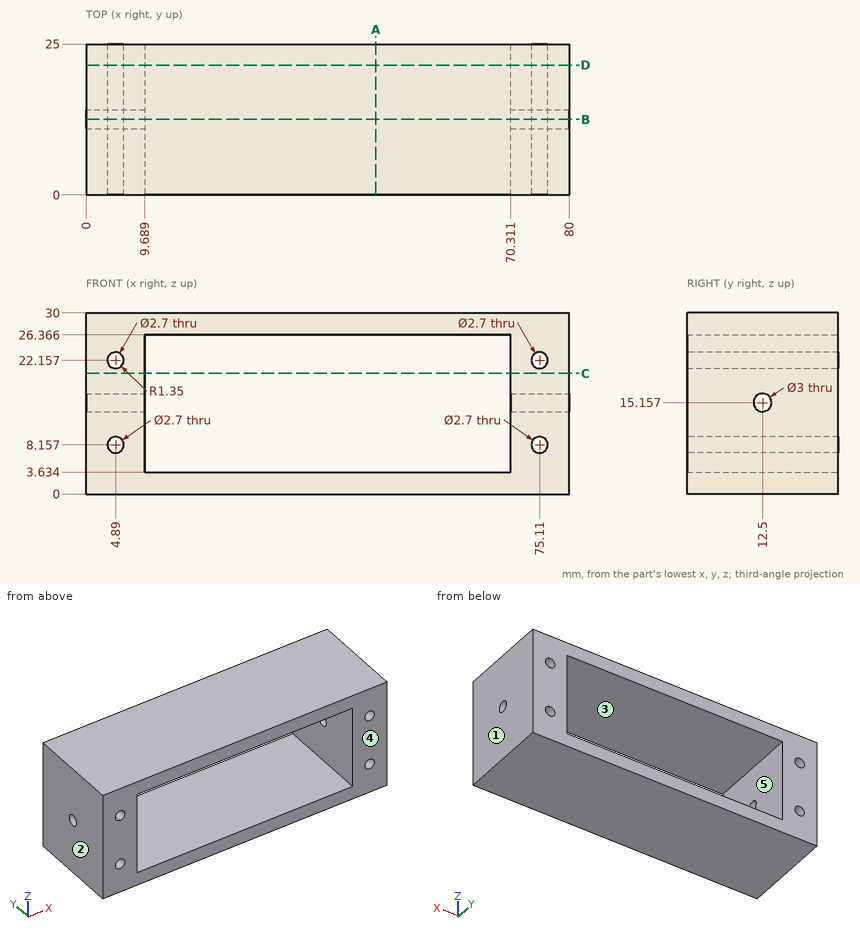
Geometry check sheet. Reference: drawing and pictorial views, mm from the part's lowest x, y, z. A direction names the side the tool comes from. Round coordinates to 2 decimals unless told otherwise and drop trailing zeros. Write each loop counter-clockwise with the first axis right and the second up, starting at its lowest first coordinate (ties: lowest second). Pieces come first, ordered by that corner, then holes. Notation, with made-up numbers: (-30, 80.5) -> (-12, 80.5) arc R25 ccw to (-12, 101.5) -> close; hole circle Ø8 at (43, 32). An arc over 180 degrees is marked (long way). Put each result on its own line as item: value.
1) Release check for a two-part mould opening along X. For the marked faces 1, 2 and 3 record: pulls with the +X half, pulls with the -X half, needs draft (parallel to the pull), parting line crosses it, or undercut.
Recorded:
face 1: pulls with the +X half
face 2: pulls with the -X half
face 3: undercut
2) Cross-section at B-B, the plane y = 12.5. Enter the section's corners in (x, z).
Recorded:
outline: (0, 0) -> (80, 0) -> (80, 13.66) -> (70.31, 13.66) -> (70.31, 3.63) -> (9.69, 3.63) -> (9.69, 13.66) -> (0, 13.66) -> close; (0, 16.66) -> (9.69, 16.66) -> (9.69, 26.37) -> (70.31, 26.37) -> (70.31, 16.66) -> (80, 16.66) -> (80, 30) -> (0, 30) -> close; hole circle Ø2.7 at (4.89, 8.16); hole circle Ø2.7 at (4.89, 22.16); hole circle Ø2.7 at (75.11, 8.16); hole circle Ø2.7 at (75.11, 22.16)
3) Thickness scan on probe 1 along X at (y, z) = (11.5, 4.5); probe 2 along Z at (x, y) = (21, 10.5); probe 3 along Y at (x, z) = (71, 16.5) (1 decimal). Record the ranges inside material, lowest first. Write a range as from..to.
Recorded:
probe 1: x = 0..9.69, 70.31..80
probe 2: z = 0..3.63, 26.37..30
probe 3: y = 0..11.8, 13.2..25
4) Cross-section at A-A, the plane x = 48. Enter the section's corners in (y, z), plus the area to 3 significant figures.
Recorded:
outline: (0, 0) -> (25, 0) -> (25, 3.63) -> (0, 3.63) -> close; (0, 26.37) -> (25, 26.37) -> (25, 30) -> (0, 30) -> close
area: 182 mm2
5) Access from +Z, -Z, +X, -X, +Y, -Y to the whole of each face (thin tool, end or side, straight path). Record for the marked faces 4 and 5.
Recorded:
face 4: +Z, -Z, +X, -X, -Y
face 5: +Y, -Y
6) Cross-section at D-D, the plane y = 21.5. Enter the section's corners in (x, z), plus the area to 3 significant figures.
Recorded:
outline: (0, 0) -> (80, 0) -> (80, 30) -> (0, 30) -> close; hole circle Ø2.7 at (4.89, 8.16); hole circle Ø2.7 at (4.89, 22.16); hole (9.69, 3.63) -> (70.31, 3.63) -> (70.31, 26.37) -> (9.69, 26.37) -> close; hole circle Ø2.7 at (75.11, 8.16); hole circle Ø2.7 at (75.11, 22.16)
area: 999 mm2
7) Cross-section at C-C, the plane z = 20. Enter the section's corners in (x, y).
Recorded:
outline: (0, 0) -> (9.69, 0) -> (9.69, 25) -> (0, 25) -> close; (70.31, 0) -> (80, 0) -> (80, 25) -> (70.31, 25) -> close
